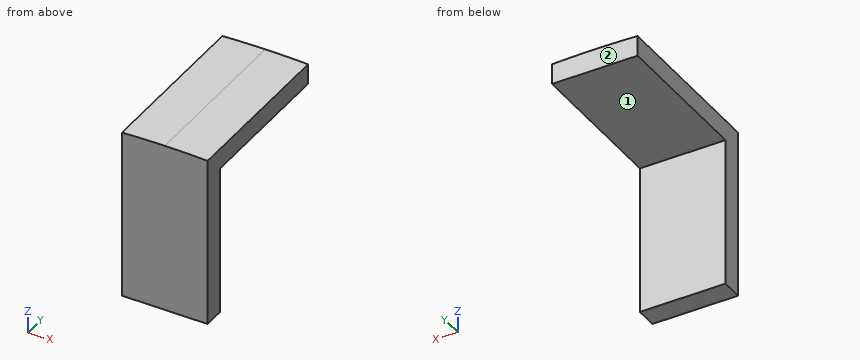
```python
from build123d import *

# Parameters (mm, degrees)
BOSS_EXTRUDE1_DEPTH = 6.35
CUT_EXTRUDE1_START  = -12.7
CUT_EXTRUDE1_DEPTH  = 12.7


# Read off the part's stored shape, not the designer's step: Cut-Extrude1
with BuildPart() as part:
    # Sketch1 → Boss-Extrude1 (new body)
    with BuildSketch(Plane(origin=(0, 0, 0), x_dir=(0, 0, -1), z_dir=(1, 0, 0))):
        Polygon((0, 0), (12.7, 0), (12.7, 1.5875), (1.5875, 1.5875), (1.5875, 12.7), (0, 12.7), align=None)
    extrude(amount=BOSS_EXTRUDE1_DEPTH)

    # Cut-Extrude1 outline → Cut-Extrude1 (cut)
    with BuildSketch(Plane(origin=(0, 12.7, 0), x_dir=(1, 0, 0), z_dir=(0, 1, 0)).offset(CUT_EXTRUDE1_START)):
        with BuildLine():
            ThreePointArc((6.35, 0.066174567), (4.762844565, 0.016545434), (3.174999586, 0))
            Line((3.174999586, 0), (6.35, 0))
            Line((6.35, 0), (6.35, 0.066174567))
        make_face()
        with BuildLine():
            ThreePointArc((3.174999586, 0), (1.587155022, 0.016545442), (0, 0.066174567))
            Line((0, 0.066174567), (0, 0))
            Line((0, 0), (3.174999586, 0))
        make_face()
    extrude(amount=CUT_EXTRUDE1_DEPTH, mode=Mode.SUBTRACT)


solid = part.part
```
The listing builds one solid part. Answer for the finished solid, in the listing's coordinates (mm). Face numbers are marked on the shaded views. A direction names the side the tool comes from. Round coordinates to 2 decimals unless told otherwise and drop trailing zeros. Write each loop counter-clockwise with the first axis right and the second up, starting at its lowest first coordinate (ties: lowest second). Pieces come first, ordered by that corner, then holes. Notation, with made-up numbers: (16, 28) -> (51, 28) arc R24 ccw to (51, 54) -> close; hole circle Ø10 at (21, -29.75). An arc over 180 degrees is marked (long way). Answer as a JSON object with one key per item and string values. Group by question number.
Q1. Which of the six approach directions +Z, -Z, +X, -X, +Y, -Y give full straight-line access (tool end or side, diameter ignored) to the marked faces 1 and 2?
Q2. Section B-B (z = -8.5) is taken. Write down the section's boundary in (x, y), plus the area to 3 significant figures.
Q3. Section C-C (x = 5.5) is taken. Write down the section's boundary in (y, z), plus the area to 3 significant figures.
Q4. Straight lines are drawn through the part: line 1 along Y through (x, z) = (1.75, -7); line 2 along Z through (x, y) = (2.75, 5). For each, find the intervals that lie inside material, in ascending order.
Q5. Each of these flat-tipped pins is pushed along its axis until it touches: pin 1 Ø1.5 at (x, y) = (1, 10.5) entering from +Z; pin 2 Ø3 at (x, y) = (4.5, 9) entering from -Z; pin 3 Ø2 at (x, z) = (1, -6.5) entering from +Y. Where does it stop, or does it pass through?
Q6. Section D-D (x = 3.5) is taken. Write down the section's boundary in (y, z).
Check values:
{
 "1": {"face 1": "-Z, +X, -X, +Y", "face 2": "+Z, -Z, +X, -X, +Y"},
 "2": {"outline": "(0, 0) -> (6.35, 0) -> (6.35, 1.59) -> (0, 1.59) -> close", "area": "10.1 mm^2"},
 "3": {"outline": "(0, -12.7) -> (1.59, -12.7) -> (1.59, -1.59) -> (12.7, -1.59) -> (12.7, -0.04) -> (0, -0.04) -> close", "area": "37.4 mm^2"},
 "4": {"line 1": "0 to 1.59", "line 2": "-1.59 to 0"},
 "5": {"pin 1": "z = -0.01", "pin 2": "z = -1.59", "pin 3": "y = 1.59"},
 "6": {"outline": "(0, -12.7) -> (1.59, -12.7) -> (1.59, -1.59) -> (12.7, -1.59) -> (12.7, 0) -> (0, 0) -> close"}
}
